```python
from build123d import *

# Parameters (mm, degrees)
F0_W        = 11.43
F0_H        = 11.43
F0_R        = 2.15265
F1_DEPTH    = 22.4125
F2_W        = 11.43
F2_H        = 11.43
F3_DEPTH    = 1.5875
F4_R        = 1.35255
F5_REACH    = 15.2565891076
F6_T1_DEPTH = 52.575
F7_R        = 2.15265
F8_DEPTH    = 196.85


# Not quite as in the source:
# - a fillet or chamfer that OpenCascade refuses, or shapes differently, is made with other operations: its cross-section is extruded or revolved along the edge and cut away or added


with BuildPart() as f1:
    # F0 (on Top) → F1 (new body)
    with BuildSketch(Plane.XY):
        Rectangle(F0_W, F0_H)
        Circle(F0_R, mode=Mode.SUBTRACT)
    extrude(amount=F1_DEPTH)

    # F2 (on face) → F3 (join)
    with BuildSketch(Plane.XY.offset(22.4125)):
        Rectangle(F2_W, F2_H)
    extrude(amount=F3_DEPTH)

    f5_end = f1.faces().sort_by_distance((-2.15265, 0, 11.20625))[0]
    # F4 (on face) → F5 (cut, up to a face of the model that its end follows)
    with BuildSketch(Plane(origin=(-5.715, 0, 0), x_dir=(0, -1, 0), z_dir=(-1, 0, 0))):
        with Locations((0, 11.20625)):
            Circle(F4_R)
    f5_long = extrude(amount=-F5_REACH, mode=Mode.PRIVATE)
    add(split(f5_long, bisect_by=f5_end, keep=Keep.ALL, mode=Mode.PRIVATE).solids().sort_by_distance((-5.715, 0, 11.20625))[0], mode=Mode.SUBTRACT)

    # F6: fillet of radius 5.715 on 4 edges, made by hand

    # F6_s2 → F6_t1 (cut)
    with BuildSketch(Plane.XY.offset(-14.2875)):
        with BuildLine():
            ThreePointArc((0, -5.715), (-4.0411152545, -4.0411152545), (-5.715, 0))
            Line((-5.715, 0), (-5.715, -5.715))
            Line((-5.715, -5.715), (0, -5.715))
        make_face()
        with BuildLine():
            ThreePointArc((0, -5.715), (4.0411152545, -4.0411152545), (5.715, 0))
            Line((5.715, 0), (5.715, -5.715))
            Line((5.715, -5.715), (0, -5.715))
        make_face()
        with BuildLine():
            ThreePointArc((-5.715, 0), (-4.0411152545, 4.0411152545), (0, 5.715))
            Line((0, 5.715), (-5.715, 5.715))
            Line((-5.715, 5.715), (-5.715, 0))
        make_face()
        with BuildLine():
            ThreePointArc((5.715, 0), (4.0411152545, 4.0411152545), (0, 5.715))
            Line((0, 5.715), (5.715, 5.715))
            Line((5.715, 5.715), (5.715, 0))
        make_face()
    extrude(amount=F6_T1_DEPTH, mode=Mode.SUBTRACT)

    # F7 (on face) → F8 (join)
    with BuildSketch(Plane.XY.offset(24)):
        Circle(F7_R)
    extrude(amount=F8_DEPTH)


solid = f1.part
```
CAD build for the part. Positions are in the model's coordinates, mm. A direction names the side the tool comes from. Coordinates: 2 decimals unless noted, no trailing zeros. Write each loop counter-clockwise with the first axis right and the second up, starting at its lowest first coordinate (ties: lowest second). Pieces come first, ordered by that corner, then holes.
(1) Cut at B-B, the plane x = 4. List the corners of the cut face in (y, z), and give its area (3 significant figures).
(2) 3-axis set-ups, long thin cutter, end or side, ignore diameter. For faces 4 (the face through (0, 0, 22.412)), 5 (the face through (-0.1, -2.5, 0)), 6 (the face through (-0.1, -2.5, 24)): which of +Z, -Z, +X, -X, +Y, -Y reach the whole face in a straight line?
(3) Two-plate mould, pull along X, no slides. Class faces 1 (the face through (0, 0, 220.85)), 2 (the face through (2.053, 0.647, 11.049)), 3 (the face through (-0.28, 2.134, 121.047)): +X half, -X half, draft (parallel to the pull), parting line (faces both ways), or undercut.
(4) Flat gauge pins, fed straight in: pin 1 (3.5 mm diameter, centred on x = 0.5, y = -1, fed in from -Z); pin 2 (5 mm diameter, centred on y = 1.5, z = 197, fed in from -X); pin 3 (2.5 mm diameter, centred on x = 0, y = 0, fed in from -Z); pin 4 (6 mm diameter, centred on x = 3, z = 66, fed in from -Y). Where does each tip first touch, or does it go through?
(5) Drill centre lines: probe 1 along Y at (x, z) = (0, 13.75) (3 decimals); probe 2 along Z at (x, y) = (-3.25, 0); probe 3 along X at (y, z) = (0.5, 17.5). Where is each one in solid material? Low to high.
(6) Cut at A-A, the plane z = 73.5. List the corners of the cut face in (x, y), and give its area (3 significant figures).
Geometry says:
1. outline: (-4.08, 0) - (4.08, 0) - (4.08, 24) - (-4.08, 24) - close
1. area: 196 mm2
2. face 4: -Z
2. face 5: -Z, +X, -X, +Y, -Y
2. face 6: +Z
3. face 1: draft
3. face 2: undercut
3. face 3: parting line
4. pin 1: stops at z = 0
4. pin 2: stops at x = -2.15
4. pin 3: stops at z = 22.41
4. pin 4: stops at y = -2.15
5. probe 1: y = -5.715 to -2.153, 2.153 to 5.715
5. probe 2: z = 0 to 9.85, 12.56 to 24
5. probe 3: x = -5.69 to -2.09, 2.09 to 5.69
6. outline: circle Ø4.31 at (0, 0)
6. area: 14.6 mm2
